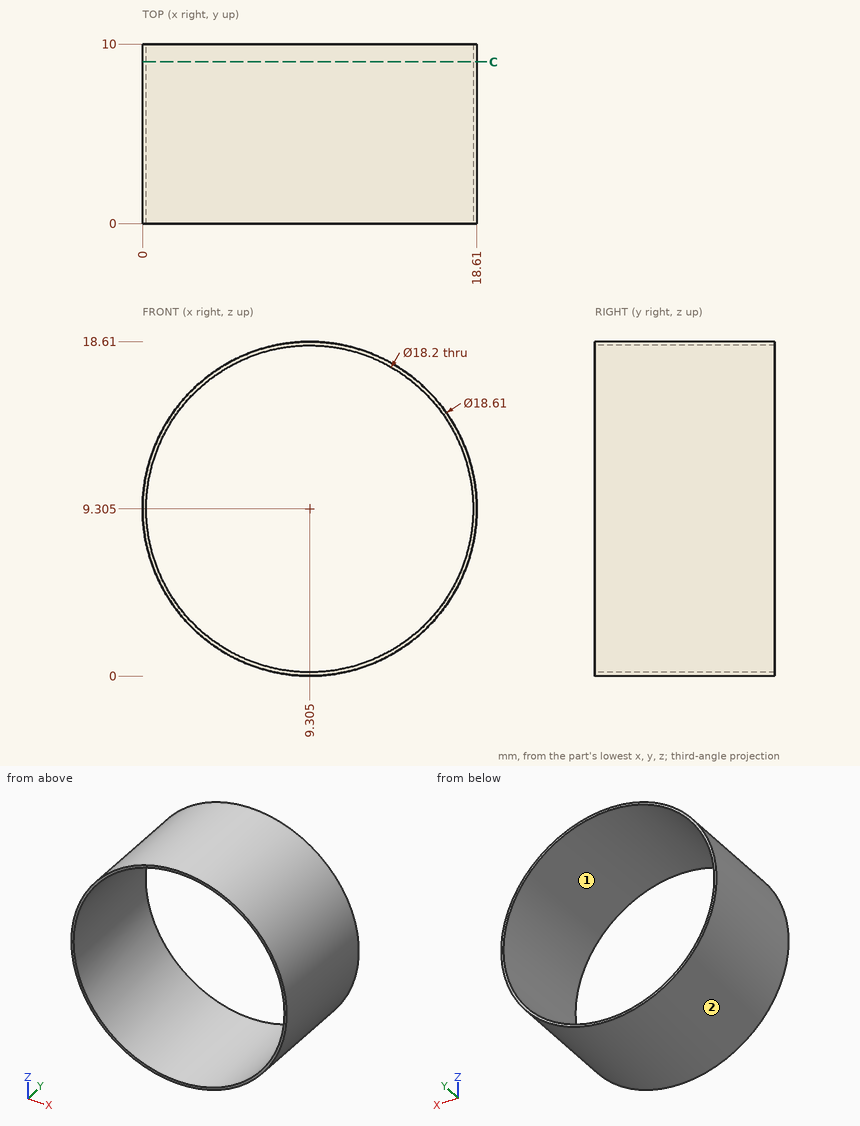
Input: dimensioned drawing with shaded views. Units: mm. Origin: part minimum x, y, z. Round coordinates to 2 decimals unless told otherwise and drop trailing zeros. Order: outer loops, then holes, each group sorted by start corner. A loop starts at its lowest first (then second) coordinate and runs counter-clockwise, first axis right, second up. Notation, with made-up numbers: (21.5, -25.75) - (59.5, -25.75) arc R16 ccw to (59.5, -11.75) - close; hole circle Ø11 at (42, 25.5). An arc over 180 degrees is marked (long way). Use CSV: the item, a comma, the result in double quotes. Start each with the question number.
Q1. Section query C-C (y = 9). Return loops of the section in (x, z) (1 decimal).
Q2. Mould query, pull axis Z, two halves, no side actions, for the marked faces 1 and 2. Classes: +Z half, -Z half, draft (parallel to the pull), parting line (faces both ways), or undercut.
Q3. Material intervals for line 1 along X through (y, z) = (5.75, 9.25) (1 decimal); line 2 along X through (y, z) = (7, 4); line 3 along Z through (x, y) = (6.5, 8.5), sorted ascending. Write a range as from..to.
Q4. First-contact query: pin 1 (2 mm diameter, centred on x = 3, y = 4, fed in from -Z); pin 2 (1.5 mm diameter, centred on x = 7.5, y = 7, fed in from -Z); pin 3 (4 mm diameter, centred on x = 3.5, z = 10, fed in from +Y); pin 4 (2 mm diameter, centred on x = 4, y = 9, fed in from +Z). Flat tips, straight axial feed; report the tip coordinate or a pass-through.
Result set:
1,outline,"circle Ø18.6 at (9.3, 9.3); hole circle Ø18.2 at (9.3, 9.3)"
2,face 1,"undercut"
2,face 2,"parting line"
3,line 1,"x = 0..0.2, 18.4..18.6"
3,line 2,"x = 1.66..1.91, 16.7..16.95"
3,line 3,"z = 0.43..0.65, 17.96..18.18"
4,pin 1,"stops at z = 1.66"
4,pin 2,"stops at z = 0.06"
4,pin 3,"passes through"
4,pin 4,"stops at z = 17.55"
